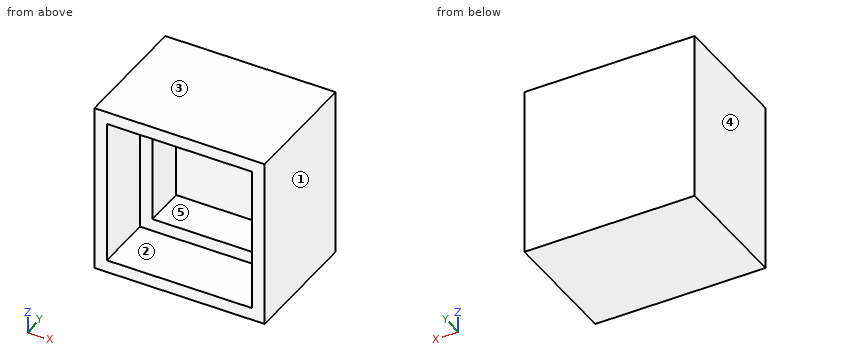
Autodesk Inventor part; units mm, degrees
ref_plane "YZ Plane" through (0, 0, 0) normal (1, 0, 0) x (0, 1, 0)
ref_plane "XZ Plane" through (0, 0, 0) normal (0, 1, 0) x (-1, 0, 0)
ref_plane "XY Plane" through (0, 0, 0) normal (0, 0, 1) x (1, 0, 0)
sketch "Sketch1" plane through (0, 0, 0) normal (0, 1, 0) x (-1, 0, 0)
  line L0 (-10.25, 10.25) -> (10.25, 10.25)
  line L1 (10.25, 10.25) -> (10.25, -10.25)
  line L2 (10.25, -10.25) -> (-10.25, -10.25)
  line L3 (-10.25, -10.25) -> (-10.25, 10.25)
  line L4 (-10.25, 10.25) -> (10.25, -10.25) construction
  line L5 (10.25, 10.25) -> (-10.25, -10.25) construction
  line L6 (-8.75, 8.75) -> (8.75, 8.75)
  line L7 (8.75, 8.75) -> (8.75, -8.75)
  line L8 (8.75, -8.75) -> (-8.75, -8.75)
  line L9 (-8.75, -8.75) -> (-8.75, 8.75)
  line L10 (-8.75, 8.75) -> (8.75, -8.75) construction
  line L11 (8.75, 8.75) -> (-8.75, -8.75) construction
  point P0 (0, 0)
  dimension "d0" = 1.5
  dimension "d1" = 20.5
extrude "Extrusion1" add sketch "Sketch1" along normal blind 7
sketch "Sketch2" plane through (0, 7, 0) normal (0, 1, 0) x (1, 0, 0)
  line L0 (10.25, -10.25) -> (-10.25, -10.25)
  line L1 (-10.25, -10.25) -> (-10.25, 10.25)
  line L2 (-10.25, 10.25) -> (10.25, 10.25)
  line L3 (10.25, 10.25) -> (10.25, -10.25)
  line L4 (10.25, -10.25) -> (-10.25, 10.25) construction
  line L5 (-10.25, -10.25) -> (10.25, 10.25) construction
  line L6 (7.25, -7.25) -> (-7.25, -7.25)
  line L7 (-7.25, -7.25) -> (-7.25, 7.25)
  line L8 (-7.25, 7.25) -> (7.25, 7.25)
  line L9 (7.25, 7.25) -> (7.25, -7.25)
  line L10 (7.25, -7.25) -> (-7.25, 7.25) construction
  line L11 (-7.25, -7.25) -> (7.25, 7.25) construction
  point P0 (0, 0)
  dimension "d4" = 3
extrude "Extrusion2" add sketch "Sketch2" along normal blind 5
sketch "Sketch3" plane through (0, 12, 0) normal (0, 1, 0) x (1, 0, 0)
  line L0 (-10.25, 10.25) -> (10.25, 10.25)
  line L1 (10.25, -10.25) -> (-10.25, -10.25)
  line L2 (-10.25, -10.25) -> (-10.25, 10.25)
  line L3 (-10.25, 10.25) -> (10.25, 10.25)
  line L4 (10.25, 10.25) -> (10.25, -10.25)
  line L5 (10.25, -10.25) -> (-10.25, 10.25) construction
  line L6 (-10.25, -10.25) -> (10.25, 10.25) construction
  point P0 (0, 0)
extrude "Extrusion3" add sketch "Sketch3" along normal blind 3
properties part number "Colorimeter_Cap"
Could you check a few things on this model? Use its own coordinates, in mm. Face numbers are marked on the shaded views. A direction names the side the tool comes from. Round coordinates to 2 decimals unless told otherwise and drop trailing zeros. Order: outer loops, then holes, each group sorted by start corner. A loop starts at its lowest first (then second) coordinate and runs counter-clockwise, first axis right, second up. Notation, with made-up numbers: M 46.25,86.5 L 97.25,86.5 A15 ccw 97.25,115.5 Z; hole C 79.25,11.25 d4. An arc over 180 degrees is marked long. One line per item, written item: value.
(1) Imagine slicing it at A-A (z = -6). Write out the boundary of the cut face in (x, y).
Ans:
outline: M -10.25,0 L -8.75,0 L -8.75,7 L -7.25,7 L -7.25,12 L 7.25,12 L 7.25,7 L 8.75,7 L 8.75,0 L 10.25,0 L 10.25,15 L -10.25,15 Z
(2) Which directions (+Z, -Z, +X, -X, +Y, -Y) give clear straight access to the entire face, cutting with the end or side of a thin tool? Please do the marked faces 1 and 2.
Ans:
face 1: +Z, -Z, +X, +Y, -Y
face 2: -Y
(3) I need wall thicknesses on line 1 along Z through (x, y) = (2, 2.5); line 2 along X through (y, z) = (11.25, -0.25). Which ranges of each line are inside material? Lowest first, please. Write a range as from..to.
Ans:
line 1: z = -10.25..-8.75, 8.75..10.25
line 2: x = -10.25..-7.25, 7.25..10.25
(4) I'm going to push a flat-ended pin straight in: P1, Ø1.5, axis at x = -4.5, z = 0.5, coming from the -Y side. Where does the tip first touch, or does it pass through?
Ans:
P1: stops at y = 12
(5) If we mould it in two halves opening along X, with no side actions, what happens to the marked faces 3, 4 and 5? For each: released by +X, released by -X, zero draft, split by the parting line, or undercut.
Ans:
face 3: zero draft
face 4: released by -X
face 5: undercut
(6) Imagine slicing it at D-D (z = 8.25). Write out the boundary of the cut face in (x, y).
Ans:
outline: M -10.25,0 L -8.75,0 L -8.75,7 L 8.75,7 L 8.75,0 L 10.25,0 L 10.25,15 L -10.25,15 Z
(7) Imagine slicing it at C-C (x = -3.5). Write out the boundary of the cut face in (y, z), and give its area (4 significant figures).
Ans:
outline: M 0,-10.25 L 15,-10.25 L 15,10.25 L 0,10.25 L 0,8.75 L 7,8.75 L 7,7.25 L 12,7.25 L 12,-7.25 L 7,-7.25 L 7,-8.75 L 0,-8.75 Z
area: 112.5 mm^2
(8) Imagine slicing it at B-B (y = 9.75). Write out the boundary of the cut face in (x, z), and give its area (3 significant figures).
Ans:
outline: M -10.25,-10.25 L 10.25,-10.25 L 10.25,10.25 L -10.25,10.25 Z; hole M -7.25,-7.25 L 7.25,-7.25 L 7.25,7.25 L -7.25,7.25 Z
area: 210 mm^2
